Autodesk Inventor part; units mm, degrees
ref_plane "YZ Plane" through (0, 0, 0) normal (1, 0, 0) x (0, 1, 0)
ref_plane "XZ Plane" through (0, 0, 0) normal (0, 1, 0) x (-1, 0, 0)
ref_plane "XY Plane" through (0, 0, 0) normal (0, 0, 1) x (1, 0, 0)
sketch "Skizze1" plane through (0, 0, 0) normal (0, 0, 1) x (1, 0, 0)
  circle A0 centre (0, 0) radius 1.5
  dimension "d0" = 3
extrude "Extrusion1" add sketch "Skizze1" along normal blind 3.5
sketch "Skizze2" plane through (0, 0, 3.5) normal (0, 0, 1) x (1, 0, 0)
  circle A0 centre (0, 0) radius 1
  dimension "d3" = 2
extrude "Extrusion2" add sketch "Skizze2" along normal blind 2.5
sketch "Skizze3" plane through (0, 0, 0) normal (0, 1, 0) x (-1, 0, 0)
  line L0 (0, 0) -> (2, 0)
  line L1 (1.5, 0) -> (-1.5, 0)
  arc A0 (-2, 0) -> (2, 0) centre (0, 1.8875) ccw
  line L2 (0, 0) -> (0, -0.8625)
  dimension "d6" = 2
  dimension "d7" = 4
  dimension "d8" = 2.75
revolve "Umdrehung1" add sketch "Skizze3" angle 360 about axis through (0, 0, 0) along (0, 0, -1)
thread "Gewinde1"
properties part number "m2mit025"
Design review of the part built by this model. Coordinates are the model's own, in mm. A direction names the side the tool comes from. Coordinates: 2 decimals unless noted, no trailing zeros. Order: outer loops, then holes, each group sorted by start corner. A loop starts at its lowest first (then second) coordinate and runs counter-clockwise, first axis right, second up.
Item 1: For line 1 (Z direction, x = 0.1, y = -0.05); line 2 (Y direction, x = 0.7, z = 5.75); line 3 (Y direction, x = -0.4, z = 2.25), list the stretches that pass through material, from the lowest coordinate up.
Item 2: Take a section at A-A, the plane x = 0. Write out the cut boundary in (y, z), then the cut area to 3 significant figures.
Item 3: Take a section at D-D, the plane x = -1.1. Write out the cut boundary in (y, z).
Item 4: Take a section at C-C, the plane z = 2.75. Write out the cut boundary in (x, y).
Item 5: For pin 1 Ø1.5 at (x, z) = (-1, 3.5) entering from +Y; pin 2 Ø2 at (x, z) = (-0.5, 1.5) entering from -Y; pin 3 Ø1.5 at (x, y) = (0.5, -1) entering from -Z, all flat-tipped, find the tip position at first contact; note any pin that passes through.
Item 6: For faces 1 (the flat face through (0, 0, 6)), 2 (the cylindrical face through (-1.5, -0.07, 1.73)), list the 3-axis set-ups (+Z, -Z, +X, -X, +Y, -Y) from which the entire face can be reached by the end or side of a thin tool; tool diameter is ignored.
The answers:
1. line 1: z = -0.86 to 6
1. line 2: y = -0.71 to 0.71
1. line 3: y = -1.45 to 1.45
2. outline: (-2, 0) arc R2.75 ccw to (2, 0) - (1.5, 0) - (1.5, 3.5) - (1, 3.5) - (1, 6) - (-1, 6) - (-1, 3.5) - (-1.5, 3.5) - (-1.5, 0) - close
2. area: 17.9 mm2
3. outline: (-1.67, 0) arc R2.52 ccw to (1.67, 0) - (1.02, 0) - (1.02, 3.5) - (-1.02, 3.5) - (-1.02, 0) - close
4. outline: circle Ø3 at (0, 0)
5. pin 1: stops at y = 1.48
5. pin 2: stops at y = -1.5
5. pin 3: stops at z = -0.84
6. face 1: +Z, +X, -X, +Y, -Y
6. face 2: +Z
